Autodesk Inventor part; units mm, degrees
ref_plane "YZ Plane" through (0, 0, 0) normal (1, 0, 0) x (0, 1, 0)
ref_plane "XZ Plane" through (0, 0, 0) normal (0, 1, 0) x (-1, 0, 0)
ref_plane "XY Plane" through (0, 0, 0) normal (0, 0, 1) x (1, 0, 0)
sketch "スケッチ1" plane through (0, 0, 0) normal (0, 0, 1) x (1, 0, 0)
  line L0 (5, -5) -> (-5, -5)
  line L1 (-5, -5) -> (-5, 5)
  line L2 (-5, 5) -> (5, 5)
  line L3 (5, 5) -> (5, -5)
  line L4 (5, -5) -> (-5, 5) construction
  line L5 (-5, -5) -> (5, 5) construction
  line L6 (4, 4) -> (-4, 4)
  line L7 (-4, 4) -> (-4, -4)
  line L8 (-4, -4) -> (4, -4)
  line L9 (4, -4) -> (4, 4)
  point P0 (0, 0)
  dimension "d0" = 10
  dimension "d1" = 10
  dimension "d2" = 1
extrude "押し出し1" add sketch "スケッチ1" along normal blind 300
sketch "スケッチ2" plane through (5, -5, 0) normal (1, 0, 0) x (0, 0, -1)
  line L0 (0, 5) -> (-300, 5)
  line L1 (0, 1) -> (-300, 1)
  line L2 (0, 0) -> (0, 10)
  line L3 (-300, 0) -> (-300, 10)
  point P0 (-195, 5)
  point P1 (-70, 5)
  point P2 (-150, 5)
  point P3 (-290, 5)
  point P4 (-10, 5)
  point P5 (-149.5, 5)
  dimension "d6" = 125
  dimension "d26" = 80
  dimension "d28" = 10
  dimension "d29" = 10
  dimension "d30" = 280
  dimension "d35" = 79.5
hole "穴1" at (5, 0, 195) at (5, 0, 70) at (5, 0, 290) at (5, 0, 10) at (5, 0, 149.5) direction (-1, 0, 0) diameter 3.2 end through all
sketch "スケッチ3" plane through (-5, 5, 0) normal (0, 1, 0) x (1, 0, 0)
  line L0 (5, 0) -> (5, -300)
  line L1 (10, -300) -> (0, -300)
  line L2 (10, 0) -> (0, 0)
  point P0 (5, -195)
  point P1 (5, -70)
  point P2 (5, -149.5)
  point P3 (5, -150)
  point P4 (5, -20)
  point P5 (5, -280)
  dimension "d15" = 125
  dimension "d27" = 80
  dimension "d31" = 20
  dimension "d32" = 20
  dimension "d33" = 79.5
  dimension "d34" = 50
hole "穴2" at (0, 5, 195) at (0, 5, 70) at (0, 5, 149.5) at (0, 5, 20) at (0, 5, 280) direction (0, -1, 0) diameter 3.2 end through all
properties part number "kaku_1010_145"
Input: part model. Units: mm. Frame: model coordinates. A direction names the side the tool comes from. Coordinates: 2 decimals unless noted, no trailing zeros. Write each loop counter-clockwise with the first axis right and the second up, starting at its lowest first coordinate (ties: lowest second). Pieces come first, ordered by that corner, then holes. Notation, with made-up numbers: (56.25, -27) -> (106.25, -27) arc R33 cw to (106.25, 2) -> close; hole circle Ø11 at (83.5, 10.25). An arc over 180 degrees is marked (long way). Answer as a JSON object with one key per item and string values.
1. First-contact query: P1, Ø4, axis at y = 0, z = 70, coming from the -X side. Flat tip, straight axial feed; report the tip coordinate or a pass-through.
Result set:
{"P1": "stops at x = -5"}
2. Access query for faces 1 (the face through (-4, 1, 148)), 2 (the face through (-4.5, 0.1, 0)). Directions: +Z, -Z, +X, -X, +Y, -Y. A direction counts if a zero-diameter tool reaches every point of the face in a straight line with its end or side. Return the directions, or none.
Result set:
{"face 1": "+Z, -Z", "face 2": "-Z, +X, -X, +Y, -Y"}
3. Material intervals for line 1 (Z direction, x = 0, y = 4.75); line 2 (Z direction, x = 4.65, y = 0); line 3 (X direction, y = -4.7, z = 195), sorted ascending. Write a range as from..to.
Result set:
{"line 1": "z = 0..18.4, 21.6..68.4, 71.6..147.9, 151.1..193.4, 196.6..278.4, 281.6..300", "line 2": "z = 0..8.4, 11.6..68.4, 71.6..147.9, 151.1..193.4, 196.6..288.4, 291.6..300", "line 3": "x = -5..-1.6, 1.6..5"}
4. Section A-A on z = 124. Return the cut outline in (x, y), then the cut area to 3 significant figures.
Result set:
{"outline": "(-5, -5) -> (5, -5) -> (5, 5) -> (-5, 5) -> close; hole (-4, -4) -> (4, -4) -> (4, 4) -> (-4, 4) -> close", "area": "36.0 mm2"}
5. Section B-B on y = 0. Count the separate pieces of the cut face and the enclosed holes in it, then the cut area to 3 significant figures.
Result set:
{"separate pieces": "12", "enclosed holes": "0", "area": "568 mm2"}
6. Mould query, pull axis Y, two halves, no side actions, for faces 3 (the face through (-4.5, 0.1, 300)), 4 (the face through (4, -1, 148)), 5 (the face through (1, -5, 148)). Classes: released by +Y, released by -Y, zero draft, split by the parting line, or undercut.
Result set:
{"face 3": "zero draft", "face 4": "undercut", "face 5": "released by -Y"}
